Read the model definition and answer for the solid it produces. Units are mm, in the model's axes. A direction names the side the tool comes from. Coordinates: 2 decimals unless noted, no trailing zeros. Order: outer loops, then holes, each group sorted by start corner. A loop starts at its lowest first (then second) coordinate and runs counter-clockwise, first axis right, second up. Notation, with made-up numbers: (42, 63) - (56, 63) arc R34 cw to (56, 101) - close; hole circle Ø9 at (-21.75, 40). An arc over 180 degrees is marked (long way). Use one line per item in the form item = value.
```python
from build123d import *

# Parameters (mm, degrees)
F0_R     = 4.7625
F1_DEPTH = 39.6875
F2_W     = 8.9802561211
F2_H     = 3.175
F3_DEPTH = 7.9375
F4_W     = 8.9802561211
F4_H     = 3.175
F5_DEPTH = 7.9375
F6_R     = 2.15265
F7_DEPTH = 7.3500001002


with BuildPart() as f1:
    # F0 (on Top) → F1 (new body)
    with BuildSketch(Plane.XY):
        Circle(F0_R)
    extrude(amount=F1_DEPTH)

    # F2 (on face) → F3 (cut)
    with BuildSketch(Plane.XY.offset(39.6875)):
        with Locations((0, -3.175)):
            Rectangle(F2_W, F2_H)
    extrude(amount=-F3_DEPTH, mode=Mode.SUBTRACT)

    # F4 (on face) → F5 (cut)
    with BuildSketch(Plane(origin=(0, 0, 0), x_dir=(1, 0, 0), z_dir=(0, 0, -1))):
        with Locations((0, 3.175)):
            Rectangle(F4_W, F4_H)
    extrude(amount=-F5_DEPTH, mode=Mode.SUBTRACT)

    # F6 (on face) → F7 (cut, up to face)
    with BuildSketch(Plane.XZ.offset(1.5875)):
        with Locations((0, 35.71875)):
            Circle(F6_R)
        with Locations((0, 3.96875)):
            Circle(F6_R)
    extrude(amount=-F7_DEPTH, mode=Mode.SUBTRACT)


solid = f1.part
```
(1) Section B-B, the plane z = 20 is taken. Write down the section's boundary in (x, y) (1 decimal).
Answer list:
outline = circle Ø9.5 at (0, 0)
(2) Section A-A, the plane x = 0 is taken. Write down the section's boundary in (y, z), then the cut area to 3 significant figures.
Answer list:
outline = (-4.76, 7.94) - (-1.59, 7.94) - (-1.59, 6.12) - (4.76, 6.12) - (4.76, 33.57) - (-1.59, 33.57) - (-1.59, 31.75) - (-4.76, 31.75) - close; (-1.59, 0) - (4.76, 0) - (4.76, 1.82) - (-1.59, 1.82) - close; (-1.59, 37.87) - (4.76, 37.87) - (4.76, 39.69) - (-1.59, 39.69) - close
area = 273 mm2
(3) Which of the six approach directions +Z, -Z, +X, -X, +Y, -Y give full straight-line access (tool end or side, diameter ignored) to faces 5 (the flat face through (0, 1, 39.688)), 6 (the flat face through (0, -3, 7.938)), 7 (the flat face through (-2, -1.588, 37))?
Answer list:
face_5 = +Z, +X, -X, +Y, -Y
face_6 = -Z, +X, -X, -Y
face_7 = +Z, +X, -X, -Y
(4) Section D-D, the plane x = -4 is taken. Write down the section's boundary in (y, z), then the cut area to 3 significant figures.
Answer list:
outline = (-2.58, 7.94) - (-1.59, 7.94) - (-1.59, 0) - (2.58, 0) - (2.58, 39.69) - (-1.59, 39.69) - (-1.59, 31.75) - (-2.58, 31.75) - close
area = 189 mm2
(5) Straight lines are drawn through the part: L1, parallel to Z at x = 0, y = 3; L2, parallel to Z at x = 1.25, y = 1.5; L3, parallel to Z at x = 0.25, y = -2. For each, find the intervals that lie inside material, in ascending order.
Answer list:
L1 = 0 to 1.82, 6.12 to 33.57, 37.87 to 39.69
L2 = 0 to 2.22, 5.72 to 33.97, 37.47 to 39.69
L3 = 7.94 to 31.75
(6) Section C-C, the plane y = 3 is taken. Write down the section's boundary in (x, z), then the cut area to 3 significant figures.
Answer list:
outline = (-3.7, 0) - (3.7, 0) - (3.7, 39.69) - (-3.7, 39.69) - close; hole circle Ø4.31 at (0, 3.97); hole circle Ø4.31 at (0, 35.72)
area = 264 mm2
(7) Given pin 1 Ø2.5 at (x, z) = (1, 3) entering from -Y; pin 2 Ø1.5 at (y, z) = (-1.5, 20) entering from -X; pin 3 Ø4 at (x, z) = (3.5, 18) entering from +Y; pin 4 Ø2.5 at (x, z) = (0, 35.72) entering from -Y, each flat-ended and moving along its own axis, determine where each tip first touches the part or whether it passes through.
Answer list:
pin_1 = -1.59
pin_2 = -4.7
pin_3 = 4.52
pin_4 = through
(8) The mould has two halves that part along Z. Classify faces 1 (the flat face through (0, -3, 31.75)), 2 (the flat face through (0, 1, 0)), 3 (the cylindrical face through (-2.15, 1.55, 35.81)), 4 (the cylindrical face through (-2.15, 1.55, 4.06)): +Z half, -Z half, draft (parallel to the pull), parting line (faces both ways), or undercut.
Answer list:
face_1 = +Z half
face_2 = -Z half
face_3 = undercut
face_4 = undercut
